Autodesk Inventor part; units mm, degrees
ref_plane "YZ Plane" through (0, 0, 0) normal (1, 0, 0) x (0, 1, 0)
ref_plane "XZ Plane" through (0, 0, 0) normal (0, 1, 0) x (-1, 0, 0)
ref_plane "XY Plane" through (0, 0, 0) normal (0, 0, 1) x (1, 0, 0)
sketch "Sketch1" plane through (0, 0, 0) normal (0, 0, 1) x (1, 0, 0)
  line L0 (0, 0) -> (2.5, 0)
  line L1 (2.5, 0) -> (2.5, 28)
  line L2 (2.5, 28) -> (-2.5, 28)
  line L3 (-2.5, 28) -> (-2.5, 0)
  circle A0 centre (0, 0) radius 8.5
  line L4 (0, 28) -> (8.5, 28) construction
  circle A1 centre (0, 28) radius 8.5
  line L5 (-8.5, 0) -> (-8.5, 28)
  line L6 (8.5, 28) -> (8.5, 0)
  line L7 (0, 28) -> (8.5, 28)
  line L8 (0, 28) -> (-8.5, 19.5)
  line L9 (0, 28) -> (12.0208, 28) construction
  line L10 (0, 0) -> (8.5, 0)
  line L11 (0, 0) -> (-8.5, 8.5)
  line L12 (0, 0) -> (12.0208, 0) construction
  dimension "d9" = 17
  dimension "d1" = 2.5
  dimension "d2" = 28
  dimension "d3" = 5
  dimension "d5" = 17
  dimension "d10" = 2.5
  dimension "d11" = 0
  dimension "d12" = 135
  dimension "d13" = 135
extrude "Extrusion1" add sketch "Sketch1" along normal blind 20 contours L11 L3 A0 L1 L0 | L1 A0 L10 | L11 A0 L3 | A0 L3 A1 L1 | L1 A1 L6 A0 | A0 L11 L5 L8 A1 L3 | A1 L3 L8 L2 L1 | L1 L7 A1 | A1 L8 L3
sketch "Sketch2" plane through (0, 0, 0) normal (0, 0, -1) x (-1, 0, 0)
  line L0 (0, 0) -> (-8.5, 0)
  line L1 (0, 0) -> (0, 8)
  circle A0 centre (0, 8) radius 2.5
  line L2 (8.5, 8.5) -> (0, 0)
  line L3 (0, 0) -> (-1.5, 0)
  line L4 (-1.5, 0) -> (-1.5, 8)
  line L5 (-1.5, 8) -> (1.5, 8)
  line L6 (1.5, 8) -> (1.5, 0)
  line L7 (1.5, 0) -> (0, 0)
  line L8 (0, 28) -> (8.5, 19.5)
  line L9 (0, 28) -> (0, 20)
  line L10 (0, 20) -> (-1.5, 20)
  line L11 (-1.5, 20) -> (-1.5, 28)
  line L12 (-8.5, 28) -> (0, 28)
  line L13 (0, 20) -> (1.5, 20)
  line L14 (1.5, 20) -> (1.5, 28)
  line L15 (1.5, 28) -> (0, 28)
  circle A1 centre (0, 20) radius 2.5
  point P0 (1.5, 45)
  point P1 (-1.5, 22)
  point P2 (1.5, 22)
  point P3 (-1.5, 6)
  point P4 (1.5, 6)
  dimension "d16" = 8
  dimension "d17" = 5
  dimension "d18" = 1.5
  dimension "d19" = 3
  dimension "d20" = 8
  dimension "d21" = 1.5
  dimension "d22" = 1.5
  dimension "d23" = 5
extrude "Extrusion2" cut sketch "Sketch2" against normal through all
fillet "Fillet1" radius 8 4 edges at (8.5, 14, 0) (8.5, 14, 20) (-8.5, 14, 0) (-8.5, 14, 20)
sketch "Sketch4" plane through (1.5, 0, 0.0627) normal (0, -1, 0) x (1, 0, 0)
  line L0 (-10, 7.9373) -> (-10, 11.9373)
  line L1 (-10, 9.9373) -> (-8, 9.9373)
  circle A0 centre (-8, 9.9373) radius 1
  point P0 (-1.5, -0.0627)
  dimension "d31" = 2
  dimension "d32" = 2
extrude "Extrusion4" cut sketch "Sketch4" against normal through all
properties part number "ring_f2"
Work out the finished part from the listing and answer in its coordinate system (mm). A direction names the side the tool comes from. Round coordinates to 2 decimals unless told otherwise and drop trailing zeros. Order: outer loops, then holes, each group sorted by start corner. A loop starts at its lowest first (then second) coordinate and runs counter-clockwise, first axis right, second up. Notation, with made-up numbers: M -31,21 L 7,21 A18 ccw 7,52 Z; hole C 63.25,9.5 d4. An arc over 180 degrees is marked long. One line per item, written item: value.
Q1. Straight lines are drawn through the part: line 1 (X direction, y = 8, z = 10.5); line 2 (X direction, y = 15.25, z = 10); line 3 (X direction, y = 17.75, z = 10). For each, find the intervals that lie inside material, in ascending order.
Derived:
line 1: -8 to -7.37, -5.63 to -2.5, 2.5 to 8.5
line 2: -8.5 to -7.5, -5.5 to 8.5
line 3: -8.5 to -7.5, -5.5 to -1.09, 1.09 to 8.5
Q2. Find section C-C on x = 2. Write down the section's boundary in (y, z).
Derived:
outline: M 0,0.14 L 6.5,0.14 L 6.5,19.86 L 0,19.86 Z; M 9.5,0.14 L 18.5,0.14 L 18.5,19.86 L 9.5,19.86 Z; M 21.5,0.14 L 28,0.14 L 28,19.86 L 21.5,19.86 Z
Q3. Find section B-B on z = 10. Write down the section's boundary in (x, y), then the cut area to 3 significant figures.
Derived:
outline: M -8.5,8.5 L -7.5,7.5 L -7.5,20.5 L -8.5,19.5 Z; M -5.5,5.5 L -1.5,1.5 L -1.5,6 A2.5 cw long 1.5,6 L 1.5,0 L 8.5,0 L 8.5,28 L 1.5,28 L 1.5,22 A2.5 cw long -1.5,22 L -1.5,26.5 L -5.5,22.5 Z
area: 303 mm²
Q4. Flat-ended cylindrical pins translate along their axes: pin 1 (4.5 mm diameter, centred on x = 0, y = 8, fed in from -Z); pin 2 (1 mm diameter, centred on y = 12, z = 14.5, fed in from +X); pin 3 (6.5 mm diameter, centred on y = 1.5, z = 8, fed in from -X); pin 4 (5 mm diameter, centred on x = 5, y = 15, fed in from +Z). Find the tip coordinate at first contact, or state that the pin passes through.
Derived:
pin 1: through
pin 2: x = 8.25
pin 3: x = -4.75
pin 4: z = 19.75
Q5. Determine the mould class of faces 1 (the face through (-0.1, 10.5, 9.9)), 2 (the face through (4, 28, 10)), 3 (the face through (-1.5, 4, 10)), 4 (the face through (0.1, 17.5, 9.9)) for opening direction Y: released by +Y, released by -Y, zero draft, split by the parting line, or undercut.
Derived:
face 1: undercut
face 2: released by +Y
face 3: zero draft
face 4: undercut
Q6. Find section D-D on y = 16. Write down the section's boundary in (x, z), then the cut area to 3 significant figures.
Derived:
outline: M -8.5,8 A8 ccw -0.5,0 L 0.5,0 A8 ccw 8.5,8 L 8.5,12 A8 ccw 0.5,20 L -0.5,20 A8 ccw -8.5,12 Z; hole C -6.5,10 d2
area: 282 mm²
Q7. For faces 5 (the face through (-6.219, 14.175, 17.594)), 6 (the face through (1.5, 3, 10)), 7 (the face through (1.5, 25, 10)), determine the directions among +Z, -Z, +X, -X, +Y, -Y from which every point of the face is accessible in a straight line to the end or side of a thin tool.
Derived:
face 5: +Z, -X, +Y, -Y
face 6: +Z, -Z, -Y
face 7: +Z, -Z, +Y
Q8. Find section A-A on y = 9.5. Write down the section's boundary in (x, z).
Derived:
outline: M -8.5,8 A8 ccw -2,0.14 L -2,19.86 A8 ccw -8.5,12 Z; M 2,0.14 A8 ccw 8.5,8 L 8.5,12 A8 ccw 2,19.86 Z; hole C -6.5,10 d2
